Geometry check sheet. Reference: the model listing, model coordinates, mm. Face numbers are marked on the shaded views. Give positions to 0.01 mm unless a question says otherwise; leave off trailing zeros. Answer as CSV lines item,"result". Start each with the question number.
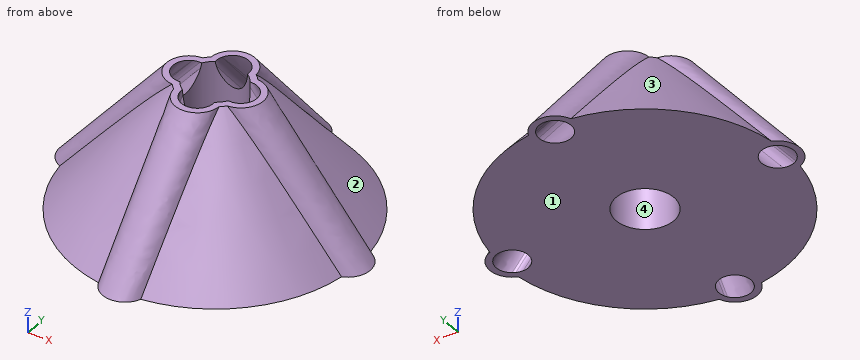
```python
from build123d import *

# Parameters (mm, degrees)
F7_COUNT  = 4
F8_COUNT  = 4
F10_R     = 0.9
F11_DEPTH = 4


with BuildPart() as f1:
    # F0 (on Front) → F1 (revolve)
    with BuildSketch(Plane.XZ):
        Polygon((-0.8, 0), (-0.8, 4), (-1.1, 4), (-4.4, 0), align=None)
    revolve(axis=Axis((0, 0, 2), (0, 0, 1)))

    # F5: sweep along a path in F4
    with BuildLine(Plane(origin=(0, 0, 0), x_dir=(0, -1, 0), z_dir=(-1, 0, 0))) as f5_path:
        Line((-4.4, 0), (-1.1, 4))
    # F2 (on face) → F5 (sweep)
    with BuildSketch(Plane.XY.offset(4)):
        with BuildLine():
            ThreePointArc((0.4582575695, 1), (0.5830784403, 0.9327483757), (0.6982120022, 0.85))
            ThreePointArc((0.6982120022, 0.85), (0, 1.5), (-0.6982120022, 0.85))
            ThreePointArc((-0.6982120022, 0.85), (-0.5830784403, 0.9327483757), (-0.4582575695, 1))
            ThreePointArc((-0.4582575695, 1), (0, 1.3), (0.4582575695, 1))
        make_face()
        with BuildLine():
            ThreePointArc((-0.4582575695, 1), (-0.5830784403, 0.9327483757), (-0.6982120022, 0.85))
            ThreePointArc((-0.6982120022, 0.85), (-0.6873150882, 0.667342661), (-0.6294528874, 0.49375))
            ThreePointArc((-0.6294528874, 0.49375), (-0.5572758185, 0.5739718304), (-0.4749588798, 0.64375))
            ThreePointArc((-0.4749588798, 0.64375), (-0.49945145, 0.823414719), (-0.4582575695, 1))
        make_face()
        with BuildLine():
            ThreePointArc((-0.6294528874, 0.49375), (0, 0.1), (0.6294528874, 0.49375))
            ThreePointArc((0.6294528874, 0.49375), (0.5572758185, 0.5739718304), (0.4749588798, 0.64375))
            ThreePointArc((0.4749588798, 0.64375), (0, 0.3), (-0.4749588798, 0.64375))
            ThreePointArc((-0.4749588798, 0.64375), (-0.5572758185, 0.5739718304), (-0.6294528874, 0.49375))
        make_face()
        with BuildLine():
            ThreePointArc((0.6294528874, 0.49375), (0.6821352583, 0.6428647417), (0.7, 0.8))
            ThreePointArc((0.7, 0.8), (0.6995528577, 0.8250159796), (0.6982120022, 0.85))
            ThreePointArc((0.6982120022, 0.85), (0.5830784403, 0.9327483757), (0.4582575695, 1))
            ThreePointArc((0.4582575695, 1), (0.4894531565, 0.9021548218), (0.5, 0.8))
            ThreePointArc((0.5, 0.8), (0.4937000303, 0.7208780685), (0.4749588798, 0.64375))
            ThreePointArc((0.4749588798, 0.64375), (0.5572758185, 0.5739718304), (0.6294528874, 0.49375))
        make_face()
    sweep(path=f5_path.line)

    # F6: sweep along a path in F4
    with BuildLine(Plane(origin=(0, 0, 0), x_dir=(0, -1, 0), z_dir=(-1, 0, 0))) as f6_path:
        Line((-4.4, 0), (-1.1, 4))
    # F2 (on face) → F6 (sweep, cut)
    with BuildSketch(Plane.XY.offset(4)):
        with BuildLine():
            ThreePointArc((-0.4582575695, 1), (0, 1.1), (0.4582575695, 1))
            ThreePointArc((0.4582575695, 1), (0, 1.3), (-0.4582575695, 1))
        make_face()
        with BuildLine():
            ThreePointArc((-0.4749588798, 0.64375), (0, 0.3), (0.4749588798, 0.64375))
            ThreePointArc((0.4749588798, 0.64375), (0, 0.8), (-0.4749588798, 0.64375))
        make_face()
        with BuildLine():
            ThreePointArc((0.5, 0.8), (0.4894531565, 0.9021548218), (0.4582575695, 1))
            ThreePointArc((0.4582575695, 1), (0, 1.1), (-0.4582575695, 1))
            ThreePointArc((-0.4582575695, 1), (-0.49945145, 0.823414719), (-0.4749588798, 0.64375))
            ThreePointArc((-0.4749588798, 0.64375), (0, 0.8), (0.4749588798, 0.64375))
            ThreePointArc((0.4749588798, 0.64375), (0.4937000303, 0.7208780685), (0.5, 0.8))
        make_face()
    f6 = sweep(path=f6_path.line, mode=Mode.SUBTRACT)

    # F7: F6 ×4 about axis
    f7_axis = Axis((0, 0, 4), (0, 0, -1))
    for i in range(1, F7_COUNT):
        add(f6.rotate(f7_axis, i * 360 / F7_COUNT), mode=Mode.SUBTRACT)


with BuildPart() as f8_1:
    # F8: instance of F1
    add(f1.part.rotate(Axis((0, 0, 0), (0, 0, 1)), 1 * 360 / F8_COUNT))


with BuildPart() as f8_2:
    # F8: instance of F1
    add(f1.part.rotate(Axis((0, 0, 0), (0, 0, 1)), 2 * 360 / F8_COUNT))


with BuildPart() as f8_3:
    # F8: instance of F1
    add(f1.part.rotate(Axis((0, 0, 0), (0, 0, 1)), 3 * 360 / F8_COUNT))


with BuildPart() as f8_2_1:
    add(f8_2.part)

    # F9: union F8_3, F1, F8_1
    add(f8_3.part)
    add(f1.part)
    add(f8_1.part)

    # F10 (on face) → F11 (cut)
    with BuildSketch(Plane(origin=(0, 0, 0), x_dir=(1, 0, 0), z_dir=(0, 0, -1))):
        Circle(F10_R)
    extrude(amount=-F11_DEPTH, mode=Mode.SUBTRACT)


solid = f8_2_1.part
```
Item 1: Depth check by flat-ended pin: pin 1 Ø2 at (x, z) = (-3, 1) entering from +Y. Enter the tip coordinate at first touch or a pass-through.
Item 2: Scan lines: line 1 along Y through (x, z) = (0, 2.6) (3 decimals); line 2 along Y through (x, z) = (0.25, 2.2); line 3 along X through (y, z) = (0, 2.3). Record each from-to range of solid material in increasing order.
Item 3: Draft check along X on the marked faces 1, 2, 3 and 4. Enter one of: pulls with the +X half, pulls with the -X half, needs draft (parallel to the pull), parting line crosses it, or undercut.
Item 4: Section check A-A on x = 0. Give the number of separate pieces and of enclosed holes in the cut face, then the cut area to 3 significant figures.
Numbers:
1,pin 1,"y = 3.49"
2,line 1,"-2.655 to -2.455, -1.455 to -0.9, 0.9 to 1.455, 2.455 to 2.655"
2,line 2,"-2.94 to -2.72, -1.85 to -0.86, 0.86 to 1.85, 2.72 to 2.94"
2,line 3,"-2.9 to -2.7, -1.7 to -0.9, 0.9 to 1.7, 2.7 to 2.9"
3,face 1,"needs draft"
3,face 2,"pulls with the +X half"
3,face 3,"pulls with the -X half"
3,face 4,"undercut"
4,separate pieces,"4"
4,enclosed holes,"0"
4,area,"10.4 mm2"
